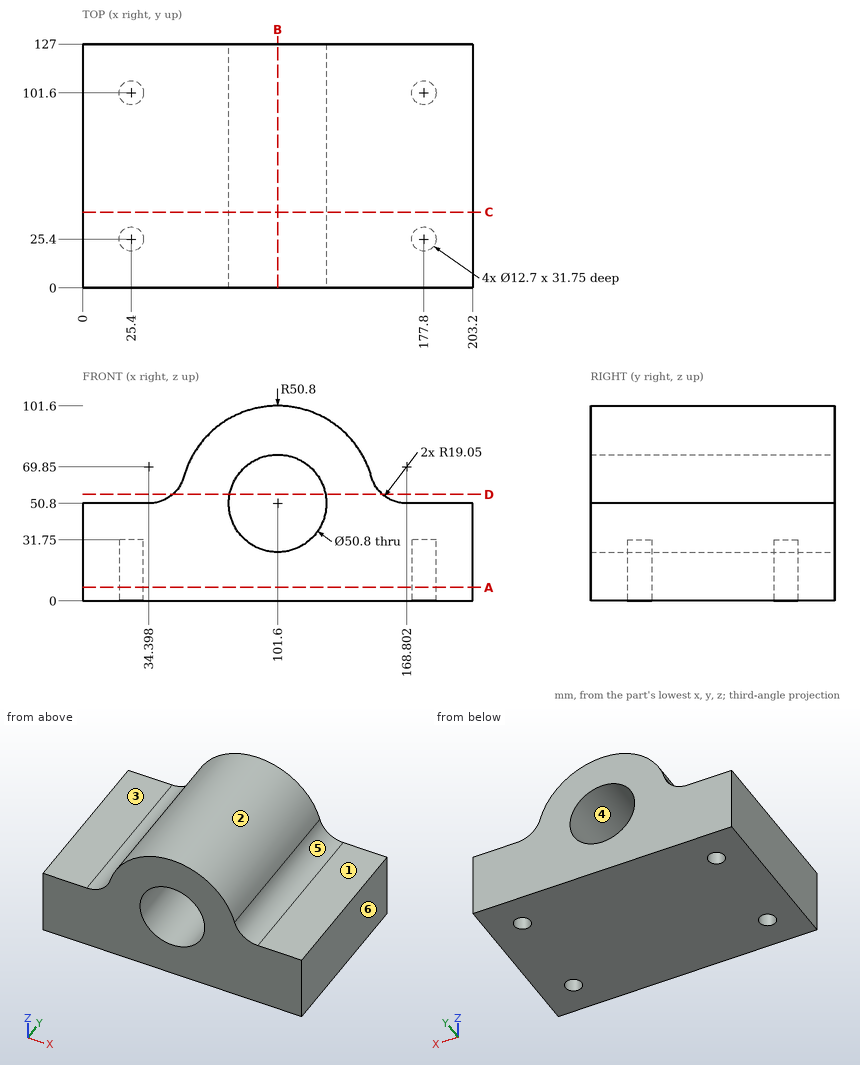
Print and shaded views of the part. All mm, measured from the part's lowest x, y and z. A direction names the side the tool comes from. Round coordinates to 2 decimals unless told otherwise and drop trailing zeros. Loops run counter-clockwise (first coordinate to the right, second up) from the corner with the lowest first, then second, coordinate; pieces in that order, holes last. Notation, with made-up numbers: (57, 59.5) -> (87, 59.5) arc R36 ccw to (87, 97.5) -> close; hole circle Ø2 at (-27.5, -39.75). An arc over 180 degrees is marked (long way). Use CSV: the item, a comma, the result in double quotes. Start each with the question number.
1) Pull direction Z, two halves, no side cores. Call the marked faces 4, 5 and 6: +Z half, -Z half, draft (parallel to the pull), parting line (faces both ways), or undercut.
2) Cut at C-C, the plane y = 39.5. Write the cut outline in (x, z).
3) Wall check: L1, parallel to Y at x = 25, z = 15; L2, parallel to X at y = 101.6, z = 20; L3, parallel to Y at x = 182.5, z = 16.5. Give the ranges that are in metal, low to high. Write a range as [from, to].
4) Which spindle directions (+Z, -Z, +X, -X, +Y, -Y) get a long thin tool onto all of the face, cutting with end or side? Do the marked faces 1, 2 and 3. Say none if no direction does.
5) Cut at B-B, the plane x = 101.6. Write the cut outline in (y, z), plus the area to 3 significant figures.
6) Cut at A-A, the plane z = 7. Write the cut outline in (x, y), plus the area to 3 significant figures.
7) Drop flat-ended pins along their axis: P1, Ø1, axis at x = 144.5, y = 91.5, coming from the +Z side; P2, Ø4, axis at x = 157, y = 102, coming from the +Z side; P3, Ø5, axis at y = 49.5, z = 57, coming from the +X side. Give the stop position or say it passes through.
8) Cut at D-D, the plane z = 55.5. Write the cut outline in (x, y), plus the area to 3 significant figures.
Determined:
1,face 4,"undercut"
1,face 5,"+Z half"
1,face 6,"draft"
2,outline,"(0, 0) -> (203.2, 0) -> (203.2, 50.8) -> (168.8, 50.8) arc R19.05 cw to (150.47, 64.65) arc R50.8 ccw to (52.73, 64.65) arc R19.05 cw to (34.4, 50.8) -> (0, 50.8) -> close; hole circle Ø50.8 at (101.6, 50.8)"
3,L1,"y = [0, 19.06], [31.74, 95.26], [107.94, 127]"
3,L2,"x = [0, 19.05], [31.75, 171.45], [184.15, 203.2]"
3,L3,"y = [0, 21.13], [29.67, 97.33], [105.87, 127]"
4,face 1,"+Z, +X, +Y, -Y"
4,face 2,"+Z, +Y, -Y"
4,face 3,"+Z, -X, +Y, -Y"
5,outline,"(0, 0) -> (127, 0) -> (127, 25.4) -> (0, 25.4) -> close; (0, 76.2) -> (127, 76.2) -> (127, 101.6) -> (0, 101.6) -> close"
5,area,"6,450 mm2"
6,outline,"(0, 0) -> (203.2, 0) -> (203.2, 127) -> (0, 127) -> close; hole circle Ø12.7 at (25.4, 25.4); hole circle Ø12.7 at (25.4, 101.6); hole circle Ø12.7 at (177.8, 25.4); hole circle Ø12.7 at (177.8, 101.6)"
6,area,"25,300 mm2"
7,P1,"stops at z = 78.78"
7,P2,"stops at z = 56.72"
7,P3,"stops at x = 157.52"
8,outline,"(46.93, 0) -> (76.64, 0) -> (76.64, 127) -> (46.93, 127) -> close; (126.56, 0) -> (156.27, 0) -> (156.27, 127) -> (126.56, 127) -> close"
8,area,"7,550 mm2"
